```python
from build123d import *

# Parameters (mm, degrees)
SKETCH_1_W       = 35
SKETCH_1_H       = 123.8
EXTRUDE_1_DEPTH  = 5
SKETCH_2_W       = 35
SKETCH_2_H       = 41
EXTRUDE_3_DEPTH  = 5
SKETCH_3_W       = 35
SKETCH_3_H       = 5
EXTRUDE_4_DEPTH  = 5
SKETCH_4_W       = 35
SKETCH_4_H       = 5
EXTRUDE_5_DEPTH  = 40
SKETCH_5_W       = 35
SKETCH_5_H       = 5
EXTRUDE_6_DEPTH  = 41
SKETCH_8_W       = 35
SKETCH_8_H       = 5
EXTRUDE_7_DEPTH  = 5
SKETCH_12_W      = 35
SKETCH_12_H      = 5
EXTRUDE_8_DEPTH  = 46
SKETCH_13_W      = 35
SKETCH_13_H      = 5
EXTRUDE_9_DEPTH  = 45
SKETCH_14_W      = 35
SKETCH_14_H      = 5
EXTRUDE_10_DEPTH = 46


with BuildPart() as part:
    # Sketch 1 → Extrude 1 (new body)
    with BuildSketch(Plane(origin=(0, 0, 0), x_dir=(1, 0, 0), z_dir=(0, 1, 0))):
        Rectangle(SKETCH_1_W, SKETCH_1_H)
    extrude(amount=EXTRUDE_1_DEPTH)



with BuildPart() as body_2:
    # Sketch 2 → Extrude 3 (new body)
    with BuildSketch(Plane(origin=(0, 0, -61.9), x_dir=(-1, 0, 0), z_dir=(0, 0, -1))):
        with Locations((0, 25.5)):
            Rectangle(SKETCH_2_W, SKETCH_2_H)
    extrude(amount=EXTRUDE_3_DEPTH)


with BuildPart() as part_1:
    add(part.part)

    add(body_2.part)  # Extrude 4 merges body 2
    # Sketch 3 → Extrude 4 (add)
    with BuildSketch(Plane(origin=(0, 0, -61.9), x_dir=(-1, 0, 0), z_dir=(0, 0, -1))):
        with Locations((0, 2.5)):
            Rectangle(SKETCH_3_W, SKETCH_3_H)
    extrude(amount=EXTRUDE_4_DEPTH)

    # Sketch 4 → Extrude 5 (add)
    with BuildSketch(Plane(origin=(0, 0, -66.9), x_dir=(-1, 0, 0), z_dir=(0, 0, -1))):
        with Locations((0, 43.5)):
            Rectangle(SKETCH_4_W, SKETCH_4_H)
    extrude(amount=EXTRUDE_5_DEPTH)

    # Sketch 5 → Extrude 6 (add)
    with BuildSketch(Plane.XZ.offset(-41)):
        with Locations((0, -104.4)):
            Rectangle(SKETCH_5_W, SKETCH_5_H)
    extrude(amount=EXTRUDE_6_DEPTH)

    # Sketch 8 → Extrude 7 (add)
    with BuildSketch(Plane.XY.offset(61.9)):
        with Locations((0, 2.5)):
            Rectangle(SKETCH_8_W, SKETCH_8_H)
    extrude(amount=EXTRUDE_7_DEPTH)

    # Sketch 12 → Extrude 8 (add)
    with BuildSketch(Plane(origin=(0, 5, 0), x_dir=(1, 0, 0), z_dir=(0, 1, 0))):
        with Locations((0, -64.4)):
            Rectangle(SKETCH_12_W, SKETCH_12_H)
    extrude(amount=EXTRUDE_8_DEPTH)

    # Sketch 13 → Extrude 9 (add)
    with BuildSketch(Plane.XY.offset(66.9)):
        with Locations((0, 48.5)):
            Rectangle(SKETCH_13_W, SKETCH_13_H)
    extrude(amount=EXTRUDE_9_DEPTH)

    # Sketch 14 → Extrude 10 (add)
    with BuildSketch(Plane.XZ.offset(-46)):
        with Locations((0, 109.4)):
            Rectangle(SKETCH_14_W, SKETCH_14_H)
    extrude(amount=EXTRUDE_10_DEPTH)


solid = part_1.part
```
For this review, take the finished solid that the model builds, in its own axes (mm). A direction names the side the tool comes from. Coordinates: 2 decimals unless noted, no trailing zeros. Write each loop counter-clockwise with the first axis right and the second up, starting at its lowest first coordinate (ties: lowest second). Pieces come first, ordered by that corner, then holes. Notation, with made-up numbers: (18.5, -23) -> (39.5, -23) arc R21 cw to (39.5, 0) -> close; hole circle Ø2 at (51, 40). An arc over 180 degrees is marked (long way). Put each result on its own line as item: value.
Q1. Take a section at A-A, the plane y = 27.5. State the section outline as (x, z) points, then the cut area to 3 significant figures.
From the geometry:
outline: (-17.5, -106.9) -> (17.5, -106.9) -> (17.5, -101.9) -> (-17.5, -101.9) -> close; (-17.5, -66.9) -> (17.5, -66.9) -> (17.5, -61.9) -> (-17.5, -61.9) -> close; (-17.5, 61.9) -> (17.5, 61.9) -> (17.5, 66.9) -> (-17.5, 66.9) -> close; (-17.5, 106.9) -> (17.5, 106.9) -> (17.5, 111.9) -> (-17.5, 111.9) -> close
area: 700 mm2
Q2. Take a section at C-C, the plane z = -32. State the section outline as (x, y) points, then the cut area to 3 significant figures.
From the geometry:
outline: (-17.5, 0) -> (17.5, 0) -> (17.5, 5) -> (-17.5, 5) -> close
area: 175 mm2
Q3. Take a section at B-B, the plane x = 7.5. State the section outline as (y, z) points, then the cut area to 3 significant figures.
From the geometry:
outline: (0, -106.9) -> (46, -106.9) -> (46, -61.9) -> (5, -61.9) -> (5, 61.9) -> (51, 61.9) -> (51, 111.9) -> (0, 111.9) -> (0, 106.9) -> (46, 106.9) -> (46, 66.9) -> (0, 66.9) -> (0, -66.9) -> (41, -66.9) -> (41, -101.9) -> (0, -101.9) -> close
area: 1,960 mm2
Q4. The part is to be moulded in two halves that separate along Z. For faces 1 (the flat face through (0, 28, 61.9)), 2 (the flat face through (-17.5, 4.8, 10.1)), 3 (the flat face through (0, 26, 111.9)), say which applies: +Z half, -Z half, draft (parallel to the pull), parting line (faces both ways), or undercut.
From the geometry:
face 1: undercut
face 2: draft
face 3: +Z half
Q5. Wall thickness on L1, parallel to Z at x = -15, y = 21; L2, parallel to Y at x = 10, z = -91.5; L3, parallel to Y at x = -10, z = -19: over which ranges is each line inside the solid? List them lowest first.
From the geometry:
L1: z = -106.9 to -101.9, -66.9 to -61.9, 61.9 to 66.9, 106.9 to 111.9
L2: y = 41 to 46
L3: y = 0 to 5
Q6. Clearance check with flat-ended pins moving along their axes: pin 1 Ø17.5 at (x, z) = (-2, -80.5) entering from -Y; pin 2 Ø12 at (x, z) = (-9, -54) entering from -Y; pin 3 Ø3 at (x, z) = (1, -55.5) entering from +Y; pin 4 Ø5 at (x, z) = (5, -83.5) entering from +Y. State where each tip first meets the part, or that it passes through.
From the geometry:
pin 1: stops at y = 41
pin 2: stops at y = 0
pin 3: stops at y = 5
pin 4: stops at y = 46
Q7. Tool access review of faces 4 (the flat face through (0, 21, -66.9)), 5 (the flat face through (0, 26, -61.9)), 6 (the flat face through (0, 46, -84)): name each direction out of +Z, -Z, +X, -X, +Y, -Y from which nothing blocks a thin tool from reaching the whole face with its end or side.
From the geometry:
face 4: +X, -X, -Y
face 5: +X, -X, +Y
face 6: -Z, +X, -X, +Y
